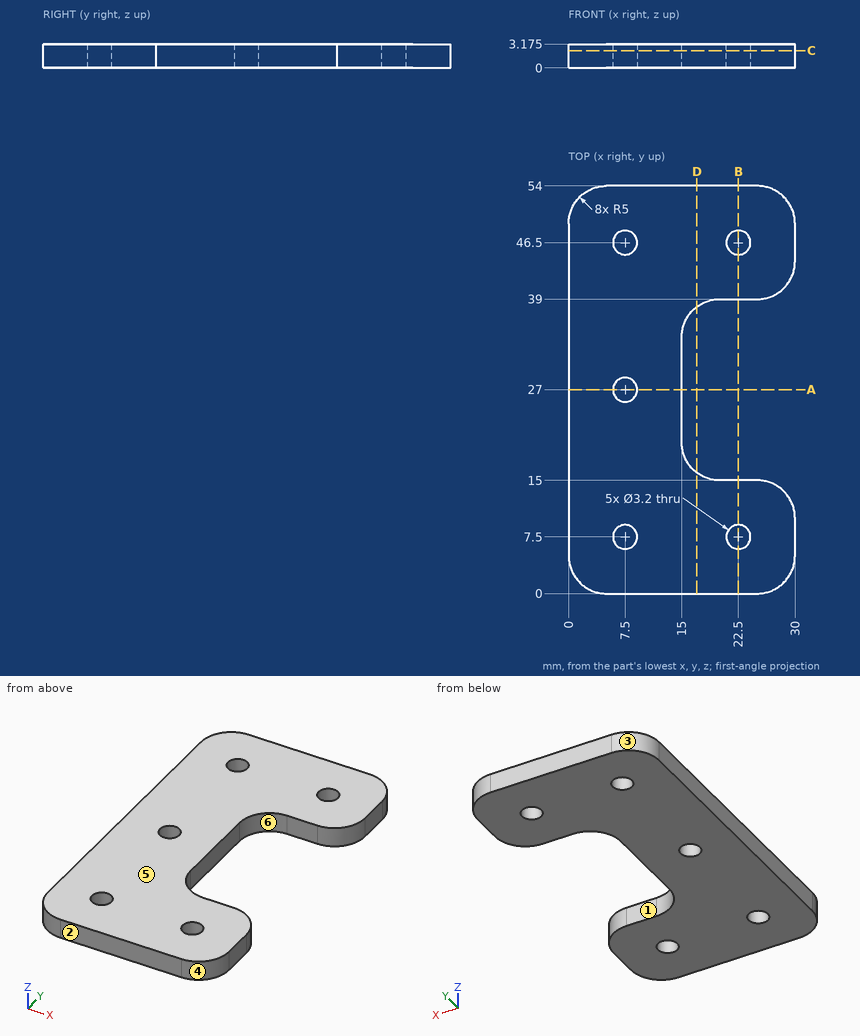
Study the drawing (mm; zero at the part's minimum x, y, z) and answer. A direction names the side the tool comes from. Give positions to 0.01 mm unless a question says otherwise; leave off trailing zeros. Order: outer loops, then holes, each group sorted by start corner. A loop starts at its lowest first (then second) coordinate and runs counter-clockwise, first axis right, second up. Notation, with made-up numbers: (65, -28.5) -> (105, -28.5) arc R17 ccw to (105, -20.5) -> close; hole circle Ø1 at (63.5, 22). An arc over 180 degrees is marked (long way). Put each result on its own line as item: value.
Item 1: For the marked faces 1 and 2, determine the directions among +Z, -Z, +X, -X, +Y, -Y from which every point of the face is accessible in a straight line to the end or side of a thin tool.
Established:
face 1: +Z, -Z, +X
face 2: +Z, -Z, +X, -X, -Y
Item 2: A cutting plane is placed at D-D on x = 17. Give the vertices of the cut face in (y, z) (3 decimals), plus the area to 3 significant figures.
Established:
outline: (0, 0) -> (16, 0) -> (16, 3.175) -> (0, 3.175) -> close; (38, 0) -> (54, 0) -> (54, 3.175) -> (38, 3.175) -> close
area: 102 mm^2
Item 3: A cutting plane is placed at B-B on x = 22.5. Give the vertices of the cut face in (y, z) (3 decimals), plus the area to 3 significant figures.
Established:
outline: (0, 0) -> (5.9, 0) -> (5.9, 3.175) -> (0, 3.175) -> close; (9.1, 0) -> (15, 0) -> (15, 3.175) -> (9.1, 3.175) -> close; (39, 0) -> (44.9, 0) -> (44.9, 3.175) -> (39, 3.175) -> close; (48.1, 0) -> (54, 0) -> (54, 3.175) -> (48.1, 3.175) -> close
area: 74.9 mm^2
Item 4: Straight lines are drawn through the part: line 1 (Y direction, x = 7.5, z = 1.8); line 2 (Y direction, x = 22.5, z = 1.7); line 3 (Y direction, x = 19, z = 1.6). For each, find the intervals that lie inside material, in ascending order.
Established:
line 1: y = 0 to 5.9, 9.1 to 25.4, 28.6 to 44.9, 48.1 to 54
line 2: y = 0 to 5.9, 9.1 to 15, 39 to 44.9, 48.1 to 54
line 3: y = 0 to 15.1, 38.9 to 54
Item 5: A cutting plane is placed at A-A on y = 27. Give the vertices of the cut face in (x, z) (3 decimals), plus the area to 3 significant figures.
Established:
outline: (0, 0) -> (5.9, 0) -> (5.9, 3.175) -> (0, 3.175) -> close; (9.1, 0) -> (15, 0) -> (15, 3.175) -> (9.1, 3.175) -> close
area: 37.5 mm^2
Item 6: Given P1, Ø5, axis at x = 22.5, y = 46.5, coming from the +Z side (3 decimals); P2, Ø1, axis at y = 14, z = 1, coming from the +X side, each flat-ended and moving along its own axis, determine where each tip first touches the part or whether it passes through.
Established:
P1: stops at z = 3.175
P2: stops at x = 28.57
Item 7: A cutting plane is placed at C-C on z = 2.3. Give the vertices of the cut face in (x, y).
Established:
outline: (0, 5) arc R5 ccw to (5, 0) -> (25, 0) arc R5 ccw to (30, 5) -> (30, 10) arc R5 ccw to (25, 15) -> (20, 15) arc R5 cw to (15, 20) -> (15, 34) arc R5 cw to (20, 39) -> (25, 39) arc R5 ccw to (30, 44) -> (30, 49) arc R5 ccw to (25, 54) -> (5, 54) arc R5 ccw to (0, 49) -> close; hole circle Ø3.2 at (7.5, 7.5); hole circle Ø3.2 at (7.5, 27); hole circle Ø3.2 at (7.5, 46.5); hole circle Ø3.2 at (22.5, 7.5); hole circle Ø3.2 at (22.5, 46.5)
Item 8: For a pull along Y with two mould halves and no side action, classify the marked faces 3, 4, 5 and 6 as released by +Y, released by -Y, zero draft, split by the parting line, or undercut.
Established:
face 3: released by +Y
face 4: released by -Y
face 5: zero draft
face 6: undercut
